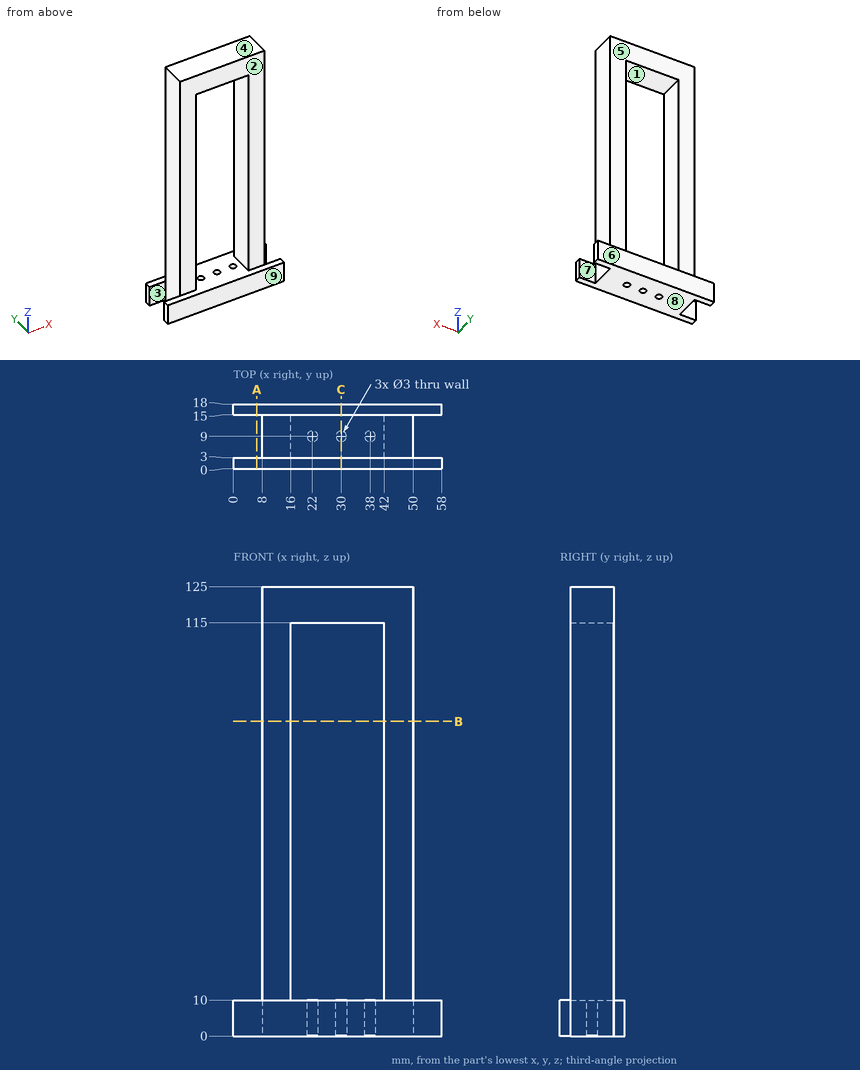
Part print with two shaded views. Sizes in mm from the minimum x, y, z corner. A direction names the side the tool comes from. Coordinates: 2 decimals unless noted, no trailing zeros. Order: outer loops, then holes, each group sorted by start corner. A loop starts at its lowest first (then second) coordinate and runs counter-clockwise, first axis right, second up. Notation, with made-up numbers: (76, 79.5) - (98, 79.5) arc R29 cw to (98, 109.5) - close; hole circle Ø7 at (-25, 54.5). An arc over 180 degrees is marked (long way). Answer in a Markdown table with one row per item.
1. Drill centre lines: L1, parallel to X at y = 9, z = 24; L2, parallel to Y at x = 30, z = 7; L3, parallel to Z at x = 18, y = 3.75. Where is each one in solid material? Low to high. Write a range as from..to.
Answer:
| item | result |
|---|---|
| L1 | 8..16, 42..50 |
| L2 | 0..7.5, 10.5..18 |
| L3 | 0..10, 115..125 |
2. Slice it at C-C, the plane x = 30. List the corners of the cut face in (y, z), then the cut area to 3 significant figures.
Answer:
| item | result |
|---|---|
| outline | (0, 0) - (7.5, 0) - (7.5, 10) - (0, 10) - close; (3, 115) - (15, 115) - (15, 125) - (3, 125) - close; (10.5, 0) - (18, 0) - (18, 10) - (10.5, 10) - close |
| area | 270 mm² |
3. 3-axis set-ups, long thin cutter, end or side, ignore diameter. For the marked faces 1, 2, 3, 4 and 5: which of +Z, -Z, +X, -X, +Y, -Y reach the whole face in a straight line?
Answer:
| item | result |
|---|---|
| face 1 | +Y, -Y |
| face 2 | +Z, +X, -X, -Y |
| face 3 | +Z, -Z, -X |
| face 4 | +Z, +X, -X, +Y, -Y |
| face 5 | +Z, +X, -X, +Y |
4. Flat gauge pins, fed straight in: P1, Ø8, axis at y = 12, z = 41.5, coming from the +X side; P2, Ø2, axis at x = 14.5, z = 26.5, coming from the +Y side; P3, Ø6.5, axis at x = 52.5, z = 3.5, coming from the -Y side; P4, Ø3.5, axis at y = 12, z = 78, coming from the -X side. Where does each tip first touch, or does it go through?
Answer:
| item | result |
|---|---|
| P1 | x = 50 |
| P2 | y = 15 |
| P3 | y = 0 |
| P4 | x = 8 |
5. Slice it at B-B, the plane z = 87.5. List the corners of the cut face in (x, y).
Answer:
| item | result |
|---|---|
| outline | (8, 3) - (16, 3) - (16, 15) - (8, 15) - close; (42, 3) - (50, 3) - (50, 15) - (42, 15) - close |
6. Slice it at A-A, the plane x = 6.5. List the corners of the cut face in (y, z).
Answer:
| item | result |
|---|---|
| outline | (0, 0) - (3, 0) - (3, 10) - (0, 10) - close; (15, 0) - (18, 0) - (18, 10) - (15, 10) - close |
7. Pull direction Y, two halves, no side cores. Call the marked faces 6, 7, 8 and 9: +Y half, -Y half, draft (parallel to the pull), parting line (faces both ways), or undercut.
Answer:
| item | result |
|---|---|
| face 6 | +Y half |
| face 7 | undercut |
| face 8 | draft |
| face 9 | -Y half |
